Check sheet for the drawn part. Datum: minimum x, y, z corner. Units: mm. A direction names the side the tool comes from. Coordinates: 2 decimals unless noted, no trailing zeros. Order: outer loops, then holes, each group sorted by start corner. A loop starts at its lowest first (then second) coordinate and runs counter-clockwise, first axis right, second up. Notation, with made-up numbers: M 68.5,83.5 L 89.5,83.5 A26 ccw 89.5,118.5 Z; hole C -8.5,-5 d1. An arc over 180 degrees is marked long. Use one line per item in the form item = value. Start each with the question number.
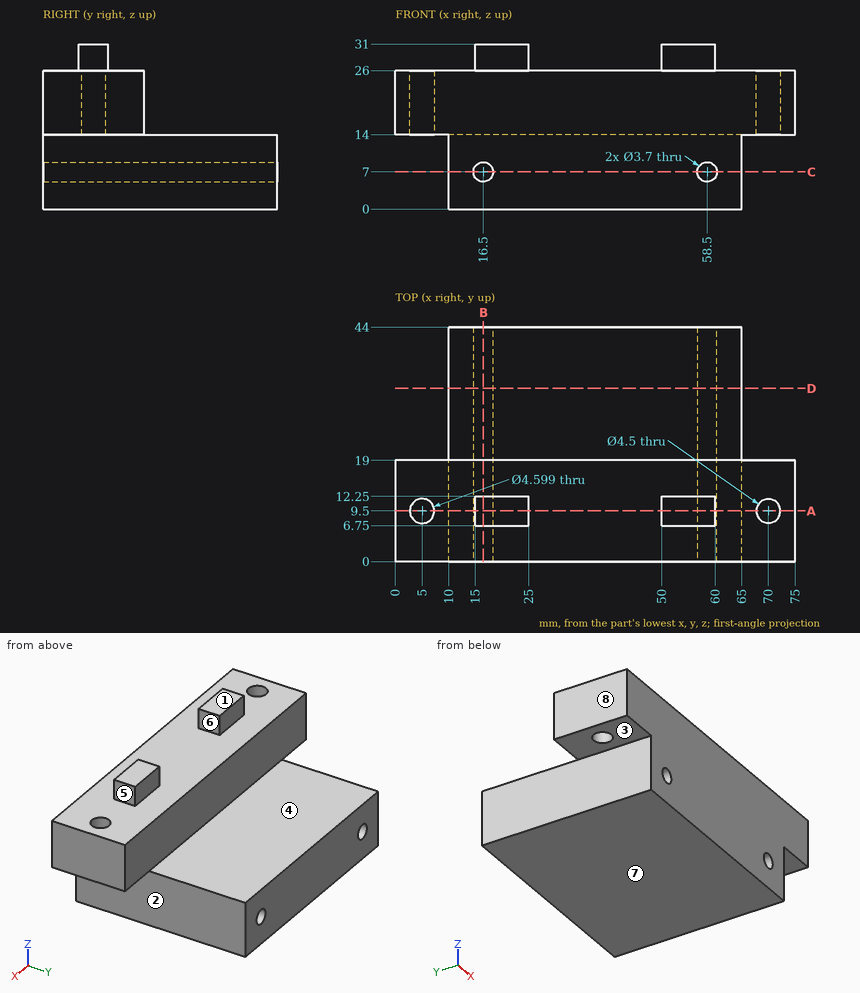
1. Cross-section at B-B on x = 16.5. Enter the section's corners in (y, z), and give its area (3 significant figures).
2. Cross-section at D-D on y = 32.5. Enter the section's corners in (x, z).
3. Cross-section at A-A on y = 9.5. Enter the section's corners in (x, z), and give its area (3 significant figures).
4. Depth check by flat-ended pin: P1, Ø1, axis at y = 18, z = 9.5, coming from the -X side; P2, Ø5, axis at x = 72, y = 11, coming from the -Z side; P3, Ø2.5, axis at y = 9.5, z = 29, coming from the +X side; P4, Ø3, axis at x = 5, y = 9.5, coming from the +Z side. Enter the tip coordinate at first touch or a pass-through.
5. Release check for a two-part mould opening along X. For the marked faces 5, 6, 7 and 8 record: pulls with the +X half, pulls with the -X half, needs draft (parallel to the pull), parting line crosses it, or undercut.
6. Cross-section at C-C on z = 7. Enter the section's corners in (x, y).
7. Tool access check on the marked faces 1, 2, 3 and 4. Record the directions out of +Z, -Z, +X, -X, +Y, -Y that give a thin tool (end or side, any length) a straight path to the whole face; none if there is none.
8. Material ranges on line 1 along X through (y, z) = (9, 22) (1 decimal); line 2 along Z through (x, y) = (16.5, 7); line 3 along Y through (x, z) = (5, 21), recorded low to high.
Final values:
q1.outline = M 0,0 L 44,0 L 44,5.15 L 0,5.15 Z; M 0,8.85 L 44,8.85 L 44,14 L 19,14 L 19,26 L 12.25,26 L 12.25,31 L 6.75,31 L 6.75,26 L 0,26 Z
q1.area = 709 mm2
q2.outline = M 10,0 L 65,0 L 65,14 L 10,14 Z; hole C 16.5,7 d3.7; hole C 58.5,7 d3.7
q3.outline = M 0,14 L 2.7,14 L 2.7,26 L 0,26 Z; M 7.3,14 L 10,14 L 10,0 L 65,0 L 65,14 L 67.75,14 L 67.75,26 L 60,26 L 60,31 L 50,31 L 50,26 L 25,26 L 25,31 L 15,31 L 15,26 L 7.3,26 Z; M 72.25,14 L 75,14 L 75,26 L 72.25,26 Z; hole C 16.5,7 d3.7; hole C 58.5,7 d3.7
q3.area = 1,640 mm2
q4.P1 = 10
q4.P2 = 14
q4.P3 = 60
q4.P4 = through
q5.face_5 = pulls with the +X half
q5.face_6 = undercut
q5.face_7 = needs draft
q5.face_8 = pulls with the -X half
q6.outline = M 10,0 L 14.65,0 L 14.65,44 L 10,44 Z; M 18.35,0 L 56.65,0 L 56.65,44 L 18.35,44 Z; M 60.35,0 L 65,0 L 65,44 L 60.35,44 Z
q7.face_1 = +Z, +X, -X, +Y, -Y
q7.face_2 = -Z, +X, +Y, -Y
q7.face_3 = -Z, -X, +Y, -Y
q7.face_4 = +Z, +X, -X, +Y
q8.line_1 = 0 to 2.8, 7.2 to 67.8, 72.2 to 75
q8.line_2 = 0 to 5.15, 8.85 to 31
q8.line_3 = 0 to 7.2, 11.8 to 19
